Geometry: see drawing. Coordinates: mm, zero at the bounding-box minimum. Coordinates: 2 decimals unless noted, no trailing zeros. Order: outer loops, then holes, each group sorted by start corner. A loop starts at its lowest first (then second) coordinate and runs counter-clockwise, first axis right, second up. Notation, with made-up numbers: (81.5, 18) -> (88.5, 18) arc R31 cw to (88.5, 49) -> close; hole circle Ø4 at (-36.5, 76.25). An arc over 180 degrees is marked (long way). Write each question's results on one line, items separated by ' | '. Start each with the question number.
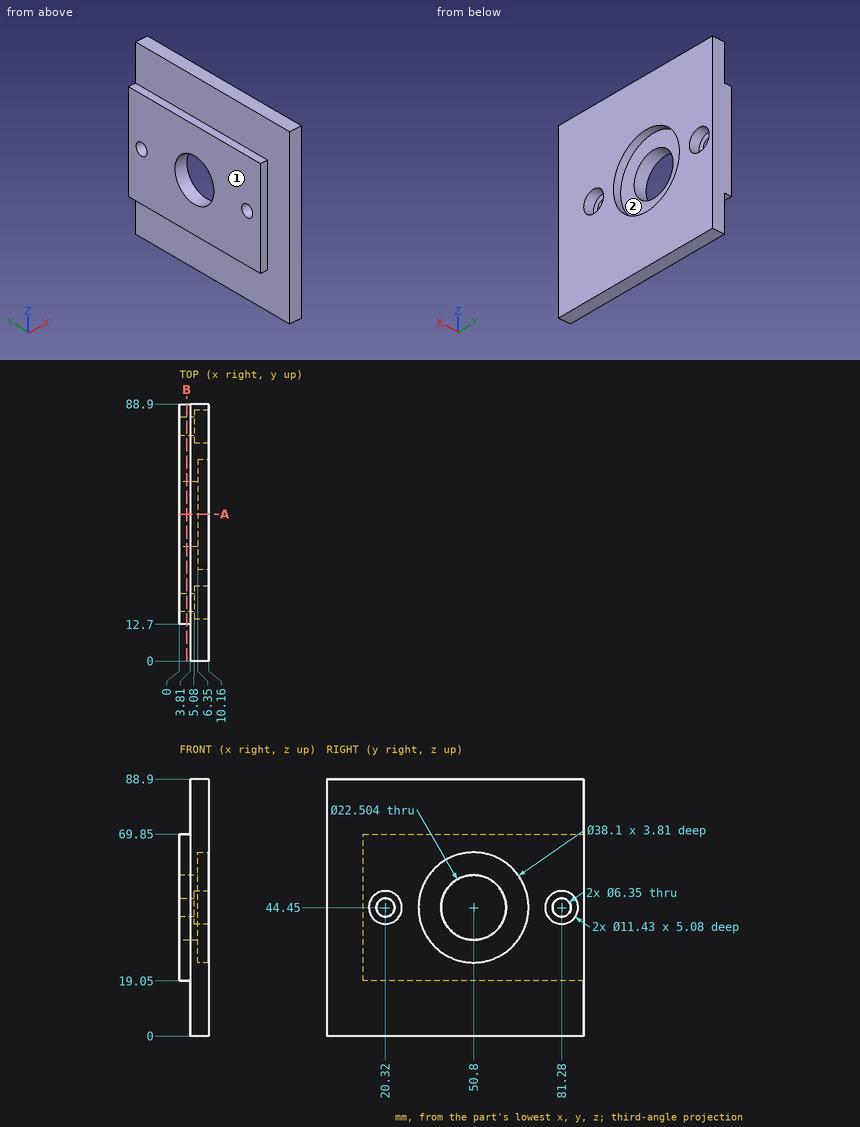
(1) Section B-B on x = 2.5. Count the separate pieces of the cut face and the enclosed holes in it, then the cut area to 3 significant figures.
(2) Line query: L1, parallel to Y at x = 1.8, z = 44.45 (1 decimal); L2, parallel to Z at x = 6.5, y = 48.5; L3, parallel to Z at x = 8.25, y = 54. Output: solid intervals per line, ascending.
(3) Section A-A on y = 50.8. Return the cut outline in (x, z), then the cut area to 3 significant figures.
(4) First-contact query: P1, Ø2, axis at x = 2, y = 58.5, coming from the +Z side; P2, Ø5.5, axis at y = 22.5, z = 43, coming from the +X side; P3, Ø2, axis at x = 2.5, y = 75, coming from the -Z side. Flat tips, straight axial feed; report the tip coordinate or a pass-through.
(5) Draft query along Z for the marked faces 1 and 2. Return one class per face: released by +Z, released by -Z, zero draft, split by the parting line, or undercut.
Results list:
1) separate pieces: 1 | enclosed holes: 3 | area: 3,410 mm²
2) L1: y = 12.7 to 17.1, 23.5 to 39.5, 62.1 to 78.1, 84.5 to 88.9 | L2: z = 0 to 25.54, 63.36 to 88.9 | L3: z = 0 to 25.67, 63.23 to 88.9
3) outline: (0, 19.05) -> (3.81, 19.05) -> (3.81, 0) -> (10.16, 0) -> (10.16, 25.4) -> (6.35, 25.4) -> (6.35, 33.2) -> (0, 33.2) -> close; (0, 55.7) -> (6.35, 55.7) -> (6.35, 63.5) -> (10.16, 63.5) -> (10.16, 88.9) -> (3.81, 88.9) -> (3.81, 69.85) -> (0, 69.85) -> close | area: 470 mm²
4) P1: stops at z = 69.85 | P2: stops at x = 5.08 | P3: stops at z = 19.05
5) face 1: zero draft | face 2: undercut
